Check sheet for the modelled part. Datum: model origin and axes. Units: mm. A direction names the side the tool comes from. Round coordinates to 2 decimals unless told otherwise and drop trailing zeros. Loops run counter-clockwise (first coordinate to the right, second up) from the corner with the lowest first, then second, coordinate; pieces in that order, holes last. Notation, with made-up numbers: (-27, 30.25) -> (-6, 30.25) arc R17 ccw to (-6, 61.25) -> close; hole circle Ø5 at (31, 81.5). An arc over 180 degrees is marked (long way). One line per item, written item: value. Start each with the question number.
1. Set-up check for faces 1 (the face through (2, 14.224, 2)), 2 (the face through (-2.23, 16.102, -3.792)): record each of +Z, -Z, +X, -X, +Y, -Y from which the full face is reachable in a straight line by a thin tool's end or side.
2. Cross-section at D-D on y = 7.25. Record the cut outline in (x, z).
3. Material ranges on L1, parallel to Y at x = 3, z = 1; L2, parallel to Z at x = 1.25, y = 5.5; L3, parallel to X at y = 10.25, z = 0.5, recorded low to high.
4. Cross-section at A-A on z = 0. Record the cut outline in (x, y).
5. Cross-section at C-C on x = 1. Record the cut outline in (y, z).
6. Cross-section at B-B on y = 14.5. Record the cut outline in (x, z), then the cut area to 3 significant figures.
Autodesk Inventor part; units mm, degrees
ref_plane "YZ Plane" through (0, 0, 0) normal (1, 0, 0) x (0, 1, 0)
ref_plane "XZ Plane" through (0, 0, 0) normal (0, 1, 0) x (-1, 0, 0)
ref_plane "XY Plane" through (0, 0, 0) normal (0, 0, 1) x (1, 0, 0)
sketch "Sketch1" plane through (0, 0, 0) normal (0, 1, 0) x (-1, 0, 0)
  circle A0 centre (0, 0) radius 2.5781
  dimension "d0" = 5.1562
extrude "Extrusion1" add sketch "Sketch1" along normal blind 14.224
sketch "Sketch2" plane through (0, 14.224, 0) normal (0, 1, 0) x (1, 0, 0)
  line L0 (0, 5.08) -> (4.3994, 2.54)
  line L1 (4.3994, 2.54) -> (4.3994, -2.54)
  line L2 (4.3994, -2.54) -> (0, -5.08)
  line L3 (0, -5.08) -> (-4.3994, -2.54)
  line L4 (-4.3994, -2.54) -> (-4.3994, 2.54)
  line L5 (-4.3994, 2.54) -> (0, 5.08)
  point P0 (0, 0)
  point P1 (0, 0)
  dimension "d3" = 5.08
extrude "Extrusion2" add sketch "Sketch2" along normal blind 3.81
sketch "Sketch3" plane through (0, 0, 0) normal (0, -1, 0) x (1, 0, 0)
  circle A0 centre (0, 0) radius 2.5781
extrude "Extrusion3" cut sketch "Sketch3" against normal blind 5.08
properties part number "Crossbeam to LS Bolt"
Taken from the geometry:
1. face 1: -Y
1. face 2: -Z, -X, +Y, -Y
2. outline: circle Ø5.16 at (0, 0)
3. L1: y = 14.22 to 18.03
3. L2: z = -2.25 to 2.25
3. L3: x = -2.53 to 2.53
4. outline: (-4.4, 14.22) -> (-2.58, 14.22) -> (-2.58, 5.08) -> (2.58, 5.08) -> (2.58, 14.22) -> (4.4, 14.22) -> (4.4, 18.03) -> (-4.4, 18.03) -> close
5. outline: (5.08, -2.38) -> (14.22, -2.38) -> (14.22, -4.5) -> (18.03, -4.5) -> (18.03, 4.5) -> (14.22, 4.5) -> (14.22, 2.38) -> (5.08, 2.38) -> close
6. outline: (-4.4, -2.54) -> (0, -5.08) -> (4.4, -2.54) -> (4.4, 2.54) -> (0, 5.08) -> (-4.4, 2.54) -> close
6. area: 67.0 mm2
